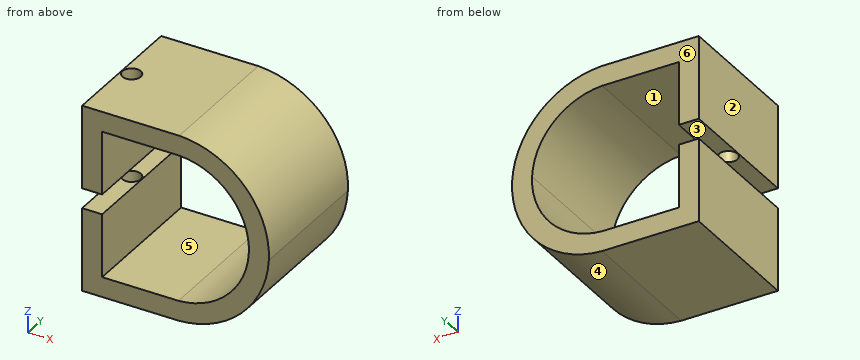
Autodesk Inventor part; units mm, degrees
ref_plane "Plan de construction2" through (-14, 20, -1.5) normal (0, 0, 1) x (1, 0, 0)
ref_plane "Plan de construction3" through (-11, 20, 1.5) normal (0, 0, -1) x (-1, 0, 0)
ref_plane "YZ Plane" through (0, 0, 0) normal (1, 0, 0) x (0, 1, 0)
sketch "Esquisse1" plane through (0, 0, 0) normal (0, 1, 0) x (-1, 0, 0)
  line L0 (11, -11) -> (11, 11)
  arc A0 (-0.5, 11) -> (-11, -0.5) centre (-0.0119, 0.0108) ccw
  arc A1 (-11, 0.5) -> (0, -11) centre (-0.0114, 0) ccw
  line L1 (11, 11) -> (-0.5, 11)
  line L2 (11, -11) -> (-0.5, -11)
  arc A2 (-0.5626, 14) -> (-13.9968, -0.6393) centre (-0.0119, 0.0108) ccw
  line L3 (-0.5626, 14) -> (14, 14)
  line L4 (14, 14) -> (14, -14)
  line L5 (14, -14) -> (-0.5, -14)
  arc A3 (-13.9968, 0.661) -> (-0.5, -14) centre (0.0221, 0.0236) ccw
  point P0 (0, 0)
  point P1 (-11, 0)
extrude "Extrusion1" add sketch "Esquisse1" along normal blind 20 contours L2 A1 A0 L1 L0 | L3 L4 L5 A3 A2
sketch "Esquisse2" plane through (0, 0, 0) normal (0, -1, 0) x (1, 0, 0)
  line L0 (13.9968, 0.661) -> (13.9968, 0.661)
  arc A0 (10.9999, 0.5232) -> (0.5, 11) centre (0.0119, 0.0108) ccw
  arc A1 (0.4408, -11) -> (10.9999, 0.5232) centre (-0.0221, 0.0236) ccw
  line L1 (0.4408, -11) -> (-11, -11)
  line L2 (-11, -11) -> (-11, 11)
  line L3 (-11, 11) -> (0.5, 11)
  point P0 (0, 0)
extrude "Extrusion2" cut sketch "Esquisse2" against normal blind 20
sketch "Esquisse3" plane through (-11, 0, 11) normal (1, 0, 0) x (0, 0, -1)
  point P0 (11, 0)
sketch "Esquisse4" plane through (0, 20, 0) normal (0, 1, 0) x (1, 0, 0)
  line L0 (-14, 1.5) -> (-11, 1.5)
  line L1 (-11, 1.5) -> (-11, -1.5)
  line L2 (-11, -1.5) -> (-14, -1.5)
  line L3 (-14, -1.5) -> (-14, 1.5)
ref_plane "Plan de construction2" through (-14, 20, -1.5) normal (0, 0, 1) x (1, 0, 0)
ref_plane "Plan de construction3" through (-11, 20, 1.5) normal (0, 0, -1) x (-1, 0, 0)
extrude "Extrusion6" cut sketch "Esquisse4" against normal through all
sketch "Esquisse7" plane through (-11, 20, 1.5) normal (0, 0, -1) x (-1, 0, 0)
  line L0 (3, 0) -> (3, -20)
  line L1 (3, 0) -> (3, -10)
  line L2 (3, -10) -> (1.5, -10)
  circle A0 centre (1.5, -10) radius 1.375
  point P0 (-11, -20)
  dimension "d46" = 10
  dimension "d47" = 1.5
  dimension "d48" = 2.75
extrude "Extrusion7" cut sketch "Esquisse7" against normal through all
sketch "Esquisse8" plane through (-14, 20, -1.5) normal (0, 0, 1) x (1, 0, 0)
  line L0 (3, 0) -> (3, -10)
  line L1 (3, -10) -> (1.5, -10)
  circle A0 centre (1.5, -10) radius 1.375
  point P0 (-11, -20)
  dimension "d51" = 10
  dimension "d52" = 1.5
  dimension "d53" = 2.75
extrude "Extrusion9" cut sketch "Esquisse8" against normal blind 3
thread "Filetage1"
thread "Filetage2"
thread "Filetage3"
properties part number "Goupille"
Input: part model. Units: mm. Frame: model coordinates. Face numbers are marked on the shaded views. A direction names the side the tool comes from. Round coordinates to 2 decimals unless told otherwise and drop trailing zeros. Loops run counter-clockwise (first coordinate to the right, second up) from the corner with the lowest first, then second, coordinate; pieces in that order, holes last. Notation, with made-up numbers: (80.25, 7) -> (90.25, 7) arc R18 cw to (90.25, 12) -> close; hole circle Ø5 at (66, -3.5). An arc over 180 degrees is marked (long way). Answer as a JSON object with one key per item and string values. Group by question number.
1) Section query A-A on x = 0. Output: boundary loops of the cut face in (y, z).
2) Section query C-C on z = -8.25. Output: boundary loops of the cut face in (x, y), plus the area to 3 significant figures.
3) Pin query (flat end, axial travel): pin 1 (1.4 mm diameter, centred on x = -12.5, y = 10.5, fed in from +Z); pin 2 (4 mm diameter, centred on y = 15.5, z = -10, fed in from +X); pin 3 (6 mm diameter, centred on y = 14, z = -9.5, fed in from +X). Return the tip coordinate at first contact, or that it passes through.
4) Draft query along Z for the marked faces 4, 5 and 6. Return one class per face: +Z half, -Z half, draft (parallel to the pull), parting line (faces both ways), or undercut.
5) Ray query, L1, parallel to Y at x = -12.5, z = 5 (3 decimals); L2, parallel to Z at x = -12.5, y = 6.75; L3, parallel to Z at x = -9.5, y = 9. Return the intervals inside material, ascending.
6) Reachability of the marked faces 1, 2 and 3 from +Z, -Z, +X, -X, +Y, -Y: full face, straight path, thin tool, end or side. Return the list, or none.
7) Section query B-B on x = -12.5. Output: boundary loops of the cut face in (y, z) (3 decimals), plus the area to 3 significant figures.
8) Section query D-D on y = 10. Output: boundary loops of the cut face in (x, z) (3 decimals).
Reply:
{
 "1": {"outline": "(0, -14) -> (20, -14) -> (20, -11) -> (0, -11) -> close; (0, 11) -> (20, 11) -> (20, 14) -> (0, 14) -> close"},
 "2": {"outline": "(-14, 0) -> (-11, 0) -> (-11, 20) -> (-14, 20) -> close; (7.28, 0) -> (11.31, 0) -> (11.31, 20) -> (7.28, 20) -> close", "area": "141 mm2"},
 "3": {"pin 1": "stops at z = -4.5", "pin 2": "stops at x = 11.49", "pin 3": "stops at x = 12.4"},
 "4": {"face 4": "-Z half", "face 5": "undercut", "face 6": "draft"},
 "5": {"L1": "y = 0 to 8.625, 11.375 to 20", "L2": "z = -14 to -1.5, 1.5 to 14", "L3": "z = -14 to -11, 11 to 14"},
 "6": {"face 1": "+Y, -Y", "face 2": "+Z, -Z, -X, +Y, -Y", "face 3": "-X, +Y, -Y"},
 "7": {"outline": "(0, -14) -> (20, -14) -> (20, -1.5) -> (11.375, -1.5) -> (11.375, -4.5) -> (8.625, -4.5) -> (8.625, -1.5) -> (0, -1.5) -> close; (0, 1.5) -> (8.625, 1.5) -> (8.625, 14) -> (0, 14) -> close; (11.375, 1.5) -> (20, 1.5) -> (20, 14) -> (11.375, 14) -> close", "area": "457 mm2"},
 "8": {"outline": "(-14, -14) -> (0.5, -14) arc R14.033 ccw to (13.996, -0.639) arc R14 ccw to (0.563, 14) -> (-11.125, 14) -> (-11.125, 1.5) -> (-11, 1.5) -> (-11, 11) -> (0.5, 11) arc R11 cw to (11, 0.523) arc R11.033 cw to (0.441, -11) -> (-11, -11) -> (-11, -1.5) -> (-11.125, -1.5) -> (-11.125, -4.5) -> (-13.875, -4.5) -> (-13.875, -1.5) -> (-14, -1.5) -> close; (-14, 1.5) -> (-13.875, 1.5) -> (-13.875, 14) -> (-14, 14) -> close"}
}
